Here's how the part is built. I have some questions about the finished solid (model axes, mm). A direction names the side the tool comes from. Coordinates: 2 decimals unless noted, no trailing zeros. Loops run counter-clockwise (first coordinate to the right, second up) from the corner with the lowest first, then second, coordinate; pieces in that order, holes last. Notation, with made-up numbers: (40.5, 65) - (59.5, 65) arc R20 ccw to (59.5, 78) - close; hole circle Ø3 at (-24.5, 67). An arc over 180 degrees is marked (long way). Use a Markdown table: item, result.
```python
from build123d import *

# Parameters (mm, degrees)
SKETCH1_R               = 15.875
SKETCH1_R_2             = 13.7668
BOSS_EXTRUDE1_DEPTH     = 203.2
CUT_EXTRUDE2_DEPTH      = 205.436472406
CUT_EXTRUDE2_DEPTH_BACK = 205.436472406
SKETCH4_R               = 2
CUT_EXTRUDE3_DEPTH      = 205.436472522
CUT_EXTRUDE3_DEPTH_BACK = 205.436472522
SKETCH3_R               = 2
CUT_EXTRUDE4_DEPTH      = 205.436472522
CUT_EXTRUDE5_DEPTH      = 205.436472522


with BuildPart() as part:
    # Sketch1 → Boss-Extrude1 (new body)
    with BuildSketch(Plane(origin=(0, 0, 0), x_dir=(1, 0, 0), z_dir=(0, 1, 0))):
        with Locations(Location((0, 0, 0), (0, 0, 270))):
            Circle(SKETCH1_R)
        with Locations(Location((0, 0, 0), (0, 0, 270))):
            Circle(SKETCH1_R_2, mode=Mode.SUBTRACT)
    extrude(amount=BOSS_EXTRUDE1_DEPTH)

    # Sketch4 → Cut-Extrude2 (cut, two sides: drawn at the far end of the back side and taken through both)
    with BuildSketch(Plane.XY.offset(-CUT_EXTRUDE2_DEPTH_BACK)):
        with Locations((0, 20.32)):
            Circle(SKETCH4_R)
    extrude(amount=CUT_EXTRUDE2_DEPTH + CUT_EXTRUDE2_DEPTH_BACK, mode=Mode.SUBTRACT)

    # Sketch3 → Cut-Extrude3 (cut, two sides: drawn at the far end of the back side and taken through both)
    with BuildSketch(Plane(origin=(0, 0, 0), x_dir=(0, 0, -1), z_dir=(1, 0, 0)).offset(-CUT_EXTRUDE3_DEPTH_BACK)):
        with Locations((0, 175.26)):
            Circle(SKETCH3_R)
    extrude(amount=CUT_EXTRUDE3_DEPTH + CUT_EXTRUDE3_DEPTH_BACK, mode=Mode.SUBTRACT)

    # Sketch5 → Cut-Extrude4 (cut, through all)
    with BuildSketch(Plane(origin=(0, 0, 0), x_dir=(0, 0, -1), z_dir=(1, 0, 0))):
        with BuildLine():
            Line((9.525, 44.45), (9.525, 0))
            Line((9.525, 0), (-9.525, 0))
            Line((-9.525, 0), (-9.525, 44.45))
            ThreePointArc((-9.525, 44.45), (0, 53.975), (9.525, 44.45))
        make_face()
    extrude(amount=CUT_EXTRUDE4_DEPTH, mode=Mode.SUBTRACT)

    # Sketch6 → Cut-Extrude5 (cut, through all)
    with BuildSketch(Plane(origin=(0, 0, 0), x_dir=(0, 0, -1), z_dir=(1, 0, 0))):
        with BuildLine():
            Line((-9.525, 0), (9.525, 0))
            Line((9.525, 0), (9.525, 12.7))
            ThreePointArc((9.525, 12.7), (0, 22.225), (-9.525, 12.7))
            Line((-9.525, 12.7), (-9.525, 0))
        make_face()
    extrude(amount=-CUT_EXTRUDE5_DEPTH, mode=Mode.SUBTRACT)


solid = part.part
```
Q1. I want a section at C-C, the plane y = 175.26. Write out the boundary of the cut face in (x, z) (3 decimals).
Check values:
| item | result |
|---|---|
| outline | (-15.749, -2) arc R15.875 ccw to (15.749, -2) - (13.621, -2) arc R13.767 cw to (-13.621, -2) - close; (-15.749, 2) - (-13.621, 2) arc R13.767 cw to (13.621, 2) - (15.749, 2) arc R15.875 ccw to start |
Q2. Will these pins go through, and if not, where does the flat tip stop? P1, Ø3, axis at x = 11.5, y = 12, coming from the -Z side; P2, Ø2, axis at x = -11, y = 6, coming from the +Z side; P3, Ø4, axis at y = 33.5, z = 3, coming from the +X side; P4, Ø3.5, axis at x = 0, y = 20.32, coming from the -Z side.
Check values:
| item | result |
|---|---|
| P1 | z = -12.33 |
| P2 | z = 12.33 |
| P3 | x = -12.83 |
| P4 | through |
Q3. I want a section at D-D, the plane y = 72.5. Write out the boundary of the cut face in (x, z) (3 decimals), then the cut area to 3 significant figures.
Check values:
| item | result |
|---|---|
| outline | circle Ø31.75 at (0, 0); hole circle Ø27.534 at (0, 0) |
| area | 196 mm^2 |
Q4. If we mould it in two halves opening along Z, with no side actions, what happens to faces 1 (the face through (14.732, 177.243, 0.26)), 2 (the face through (-15.497, 100.178, -3.441)), 3 (the face through (13, 203.2, -5))? For each: pulls with the +Z half, pulls with the -Z half, needs draft (parallel to the pull), parting line crosses it, or undercut.
Check values:
| item | result |
|---|---|
| face 1 | undercut |
| face 2 | parting line crosses it |
| face 3 | needs draft |
Q5. I want a section at B-B, the plane x = 0. Write out the boundary of the cut face in (y, z) (3 decimals), then the cut area to 3 significant figures.
Check values:
| item | result |
|---|---|
| outline | (0, -15.875) - (18.32, -15.875) - (18.32, -13.767) - (0, -13.767) - close; (0, 13.767) - (18.32, 13.767) - (18.32, 15.875) - (0, 15.875) - close; (22.32, -15.875) - (203.2, -15.875) - (203.2, -13.767) - (22.32, -13.767) - close; (22.32, 13.767) - (203.2, 13.767) - (203.2, 15.875) - (22.32, 15.875) - close |
| area | 840 mm^2 |
Q6. I want a section at A-A, the plane z = 0. Write out the boundary of the cut face in (x, y) (3 decimals).
Check values:
| item | result |
|---|---|
| outline | (-15.875, 22.225) - (-13.767, 22.225) - (-13.767, 173.26) - (-15.875, 173.26) - close; (-15.875, 177.26) - (-13.767, 177.26) - (-13.767, 203.2) - (-15.875, 203.2) - close; (13.767, 53.975) - (15.875, 53.975) - (15.875, 173.26) - (13.767, 173.26) - close; (13.767, 177.26) - (15.875, 177.26) - (15.875, 203.2) - (13.767, 203.2) - close |
Q7. Please list where these lines run through material, in increasing order: L1, parallel to X at y = 70.5, z = 0 (3 decimals); L2, parallel to X at y = 85, z = 1; L3, parallel to Y at x = 14.45, z = 0 (3 decimals). Write a range as from..to.
Check values:
| item | result |
|---|---|
| L1 | -15.875..-13.767, 13.767..15.875 |
| L2 | -15.84..-13.73, 13.73..15.84 |
| L3 | 53.975..173.26, 177.26..203.2 |
Q8. Which directions (+Z, -Z, +X, -X, +Y, -Y) give clear straight access to the entire face, cutting with the end or side of a thin tool? Please do faces 4 (the face through (14.185, 53.973, 0.209)), 5 (the face through (-1, 0, 14)).
Check values:
| item | result |
|---|---|
| face 4 | +X, -Y |
| face 5 | +Z, -Z, +X, -X, -Y |
